Part model, mm, in its own coordinate system. A direction names the side the tool comes from. Give positions to 0.01 mm unless a question says otherwise; leave off trailing zeros. Loops run counter-clockwise (first coordinate to the right, second up) from the corner with the lowest first, then second, coordinate; pieces in that order, holes last. Notation, with made-up numbers: M -0.5,-3.75 L 7.5,-3.75 A29 cw 7.5,30.25 Z; hole C 19,-28.5 d6. An arc over 180 degrees is marked long. Answer in a Markdown table with one row per item.
from build123d import *

# Parameters (mm, degrees)
F1_DEPTH = 44
F3_DEPTH = 904


with BuildPart() as f1:
    # F0 (on Front) → F1 (new body)
    with BuildSketch(Plane.XZ):
        Polygon((-22, -25), (-22, 0), (-750, 0), (-750, -25), (-634.642857, -50), (-760, -700), (-730, -700), (-583.721499, -50), (0, -50), (583.721499, -50), (730, -700), (760, -700), (634.642857, -50), (750, -25), (750, 0), (22, 0), (22, -25), (0, -25), align=None)
    extrude(amount=F1_DEPTH)

    # F2 (on Right) → F3 (cut, symmetric)
    with BuildSketch(Plane.YZ):
        Polygon((0, -700), (0, -50), (-7, -700), align=None)
        Polygon((-44, -700), (-37, -700), (-44, -50), align=None)
    extrude(amount=F3_DEPTH, both=True, mode=Mode.SUBTRACT)


solid = f1.part
(1) Pin check, flat tips, straight feed: pin 1 Ø7.5 at (y, z) = (-18, -11) entering from -X; pin 2 Ø8 at (y, z) = (-17, -97.5) entering from +X (3 decimals); pin 3 Ø1.5 at (x, y) = (4.5, -15) entering from +Z. Stop position of each tip, or through.
Recorded:
| item | result |
|---|---|
| pin 1 | stops at x = -750 |
| pin 2 | stops at x = 644.575 |
| pin 3 | stops at z = -25 |
(2) Saw through at B-B (y = -25). Write the cut outline in (x, z), plus the area to 3 significant figures.
Recorded:
| item | result |
|---|---|
| outline | M -760,-700 L -730,-700 L -583.72,-50 L 583.72,-50 L 730,-700 L 760,-700 L 634.64,-50 L 750,-25 L 750,0 L 22,0 L 22,-25 L -22,-25 L -22,0 L -750,0 L -750,-25 L -634.64,-50 Z |
| area | 124,000 mm^2 |
(3) Saw through at A-A (z = -120). Write the cut outline in (x, y), plus the area to 3 significant figures.
Recorded:
| item | result |
|---|---|
| outline | M -648.14,-43.25 L -599.47,-43.25 L -599.47,-0.75 L -648.14,-0.75 Z; M 599.47,-43.25 L 648.14,-43.25 L 648.14,-0.75 L 599.47,-0.75 Z |
| area | 4,140 mm^2 |
(4) Drill centre lines: line 1 along Z through (x, y) = (-422, -40); line 2 along X through (y, z) = (-22.5, -426); line 3 along X through (y, z) = (-36, -196.5). Where is each one in solid material? Low to high.
Recorded:
| item | result |
|---|---|
| line 1 | z = -50 to 0 |
| line 2 | x = -707.16 to -668.34, 668.34 to 707.16 |
| line 3 | x = -662.9 to -616.69, 616.69 to 662.9 |
(5) Which spindle directions (+Z, -Z, +X, -X, +Y, -Y) get a long thin tool onto all of the face, cutting with end or side? Do faces 1 (the face through (0, -22, -25)), 2 (the face through (698.2, -21.69, -379.55)), 3 (the face through (-8, -22, -50)). Say none if no direction does.
Recorded:
| item | result |
|---|---|
| face 1 | +Z, +Y, -Y |
| face 2 | +X, +Y, -Y |
| face 3 | -Z, +Y, -Y |
(6) Pull direction X, two halves, no side cores. Call faces 4 (the face through (-696.444, -21.692, -370.45)), 5 (the face through (655.837, -21.692, -370.45)), 6 (the face through (-10, 0, -30)): +X half, -X half, draft (parallel to the pull), parting line (faces both ways), or undercut.
Recorded:
| item | result |
|---|---|
| face 4 | -X half |
| face 5 | undercut |
| face 6 | draft |
(7) Saw through at C-C (x = 651). Write the cut outline in (y, z).
Recorded:
| item | result |
|---|---|
| outline | M -44,-46.46 L 0,-46.46 L 0,0 L -44,0 Z; M -43.09,-134.81 L -40.78,-348.96 L -3.22,-348.96 L -0.91,-134.81 Z |
(8) Saw through at D-D (x = -607.5). Write the cut outline in (y, z).
Recorded:
| item | result |
|---|---|
| outline | M -44,-50 L -42.86,-155.66 L -1.14,-155.66 L 0,-50 L 0,0 L -44,0 Z |
